```python
from build123d import *

# Parameters (mm, degrees)
SKETCH1_R           = 1.5
SKETCH1_R_2         = 12.5
BOSS_EXTRUDE1_DEPTH = 5


with BuildPart() as part:
    # Sketch1 → Boss-Extrude1 (new body)
    with BuildSketch(Plane(origin=(0, 0, 0), x_dir=(1, 0, 0), z_dir=(0, 1, 0))):
        with BuildLine():
            Line((-75, -75), (65, -75))
            ThreePointArc((65, -75), (72.071067812, -72.071067812), (75, -65))
            Line((75, -65), (75, 65))
            ThreePointArc((75, 65), (72.071067812, 72.071067812), (65, 75))
            Line((65, 75), (-75, 75))
            Line((-75, 75), (-97.913420794, 18.506857518))
            ThreePointArc((-97.913420794, 18.506857518), (-98.351985938, 17.031769181), (-98.5, 15.5))
            Line((-98.5, 15.5), (-98.5, -15.5))
            ThreePointArc((-98.5, -15.5), (-98.351985938, -17.031769181), (-97.913420794, -18.506857518))
            Line((-97.913420794, -18.506857518), (-75, -75))
        make_face()
        with Locations(Location((-90.5, 15.5, 0), (0, 0, 270))):
            Circle(SKETCH1_R, mode=Mode.SUBTRACT)
        with Locations(Location((-90.5, -15.5, 0), (0, 0, 270))):
            Circle(SKETCH1_R, mode=Mode.SUBTRACT)
        with Locations(Location((-59.5, -15.5, 0), (0, 0, 270))):
            Circle(SKETCH1_R, mode=Mode.SUBTRACT)
        with Locations(Location((-59.5, 15.5, 0), (0, 0, 270))):
            Circle(SKETCH1_R, mode=Mode.SUBTRACT)
        with Locations(Location((-75, 0, 0), (0, 0, 270))):
            Circle(SKETCH1_R_2, mode=Mode.SUBTRACT)
        with Locations(Location((-65, 65, 0), (0, 0, 270))):
            Circle(SKETCH1_R, mode=Mode.SUBTRACT)
        with Locations(Location((65, 65, 0), (0, 0, 270))):
            Circle(SKETCH1_R, mode=Mode.SUBTRACT)
        with Locations(Location((65, -65, 0), (0, 0, 270))):
            Circle(SKETCH1_R, mode=Mode.SUBTRACT)
        with Locations(Location((-65, -65, 0), (0, 0, 270))):
            Circle(SKETCH1_R, mode=Mode.SUBTRACT)
        with Locations(Location((0, 0, 0), (0, 0, 270))):
            Circle(SKETCH1_R, mode=Mode.SUBTRACT)
    extrude(amount=BOSS_EXTRUDE1_DEPTH)


solid = part.part
```
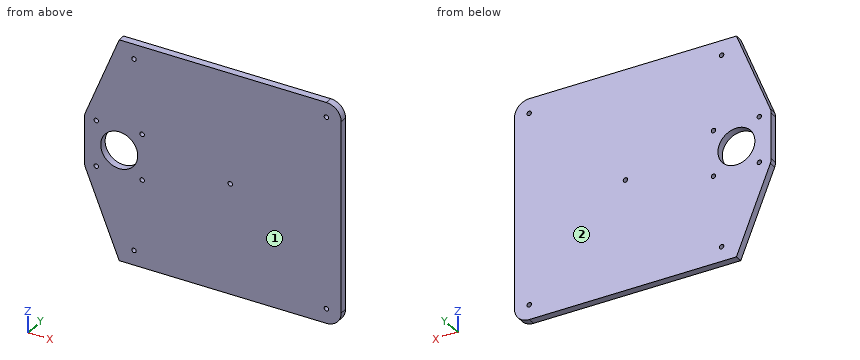
Design review of the part built by this model. Coordinates are the model's own, in mm. Face numbers are marked on the shaded views. Give positions to 0.01 mm unless a question says otherwise; leave off trailing zeros. Order: outer loops, then holes, each group sorted by start corner. A loop starts at its lowest first (then second) coordinate and runs counter-clockwise, first axis right, second up. Notation, with made-up numbers: (8, 0) - (66, 0) arc R12 cw to (66, 9) - close; hole circle Ø5 at (-35, -32.5). An arc over 180 degrees is marked (long way). Use a Markdown table: item, result. Add a question column.
(1) Clearance check with a flat-ended pin moving along its axis: P1, Ø4, axis at x = -59.5, z = -15.5, coming from the +Y side. State where the tip first meets the part, or that it passes through.
(2) Mouldability with a two-part tool opening along Y and no side actions: class the marked faces 1 and 2 as +Y half, -Y half, draft (parallel to the pull), parting line (faces both ways), or undercut.
(3) Add section B-B on y = 3.1. Give the number of separate pieces and of enclosed holes in the cut face, then the cut area to 3 significant figures.
(4) Wall thickness on probe 1 along X at (y, z) = (1.65, 0); probe 2 along X at (y, z) = (3.9, 15.5); probe 3 along Z at (x, y) = (-64.5, 2.95): over which ranges is each line inside the solid? List them lowest first. Write a range as [from, to].
(5) Add section A-A on z = 10. Give the boundary of the cut face in (x, y).
(6) Add section D-D on z = 53.5. Give the boundary of the cut face in (x, y), then the cut area to 3 significant figures.
(7) Add section C-C on z = -56. Give the boundary of the cut face in (x, y).
Report:
| question | item | result |
|---|---|---|
| 1 | P1 | stops at y = 5 |
| 2 | face 1 | -Y half |
| 2 | face 2 | +Y half |
| 3 | separate pieces | 1 |
| 3 | enclosed holes | 10 |
| 3 | area | 24,100 mm² |
| 4 | probe 1 | x = [-98.5, -87.5], [-62.5, -1.5], [1.5, 75] |
| 4 | probe 2 | x = [-98.5, -92], [-89, -61], [-58, 75] |
| 4 | probe 3 | z = [-75, -66.41], [-63.59, -6.78], [6.78, 63.59], [66.41, 75] |
| 5 | outline | (-98.5, 0) - (-82.5, 0) - (-82.5, 5) - (-98.5, 5) - close; (-67.5, 0) - (75, 0) - (75, 5) - (-67.5, 5) - close |
| 6 | outline | (-83.72, 0) - (75, 0) - (75, 5) - (-83.72, 5) - close |
| 6 | area | 794 mm² |
| 7 | outline | (-82.71, 0) - (75, 0) - (75, 5) - (-82.71, 5) - close |
